from build123d import *

# Parameters (mm, degrees)
SKETCH1_R           = 17.5
BOSS_EXTRUDE1_DEPTH = 40


with BuildPart() as part:
    # Sketch1 → Boss-Extrude1 (new body)
    with BuildSketch(Plane.XY):
        Circle(SKETCH1_R)
        with BuildLine():
            ThreePointArc((-13.167433825, 7.184614567), (-13.858192988, 5.740251485), (-14.391071429, 4.230492068))
            ThreePointArc((-14.391071429, 4.230492068), (-12.25, 0), (-14.391071429, -4.230492068))
            ThreePointArc((-14.391071429, -4.230492068), (-13.858192988, -5.740251485), (-13.167433825, -7.184614567))
            ThreePointArc((-13.167433825, -7.184614567), (-8.66205807, -8.66205807), (-7.184614567, -13.167433825))
            ThreePointArc((-7.184614567, -13.167433825), (-5.740251485, -13.858192988), (-4.230492068, -14.391071429))
            ThreePointArc((-4.230492068, -14.391071429), (0, -12.25), (4.230492068, -14.391071429))
            ThreePointArc((4.230492068, -14.391071429), (5.740251485, -13.858192988), (7.184614567, -13.167433825))
            ThreePointArc((7.184614567, -13.167433825), (8.66205807, -8.66205807), (13.167433825, -7.184614567))
            ThreePointArc((13.167433825, -7.184614567), (13.858192988, -5.740251485), (14.391071429, -4.230492068))
            ThreePointArc((14.391071429, -4.230492068), (12.25, 0), (14.391071429, 4.230492068))
            ThreePointArc((14.391071429, 4.230492068), (13.858192988, 5.740251485), (13.167433825, 7.184614567))
            ThreePointArc((13.167433825, 7.184614567), (8.66205807, 8.66205807), (7.184614567, 13.167433825))
            ThreePointArc((7.184614567, 13.167433825), (5.740251485, 13.858192988), (4.230492068, 14.391071429))
            ThreePointArc((4.230492068, 14.391071429), (0, 12.25), (-4.230492068, 14.391071429))
            ThreePointArc((-4.230492068, 14.391071429), (-5.740251485, 13.858192988), (-7.184614567, 13.167433825))
            ThreePointArc((-7.184614567, 13.167433825), (-8.66205807, 8.66205807), (-13.167433825, 7.184614567))
        make_face(mode=Mode.SUBTRACT)
    extrude(amount=BOSS_EXTRUDE1_DEPTH)


solid = part.part
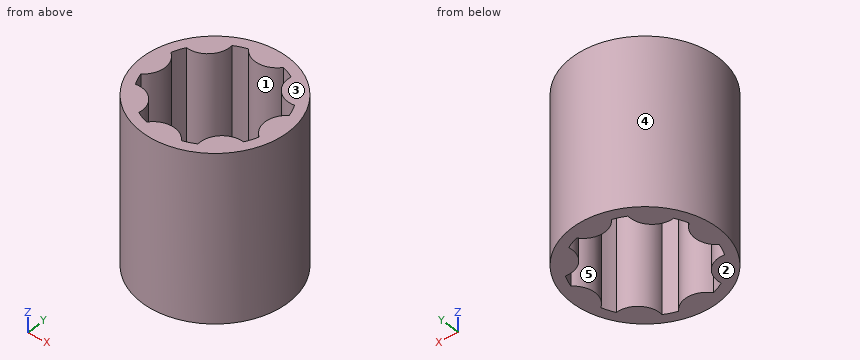
The model under review builds one solid part; all positions refer to its coordinate system, in mm. Face numbers are marked on the shaded views. A direction names the side the tool comes from. Give positions to 0.01 mm unless a question says otherwise; leave off trailing zeros. Write each loop counter-clockwise with the first axis right and the second up, starting at its lowest first coordinate (ties: lowest second). Pieces come first, ordered by that corner, then holes.
1. For P1, Ø2, axis at y = -7.5, z = 31, coming from the -X side; P2, Ø1.5, axis at y = 11, z = 16.5, coming from the -X side; P3, Ø6, axis at y = -8, z = 33.5, coming from the +X side, all flat-tipped, find the tip position at first contact; note any pin that passes through.
2. Add section D-D, the plane y = 15.5. Write out the cut boundary in (x, z).
3. Wall thickness on L1, parallel to Y at x = 13, z = 16; L2, parallel to Y at x = -10, z = 12; L3, parallel to X at y = -4.5, z = 36: over which ranges is each line inside the solid? List them lowest first.
4. Add section B-B, the plane y = 0. Write out the cut boundary in (x, z).
5. Tool access review of the marked faces 1 and 2: name each direction out of +Z, -Z, +X, -X, +Y, -Y from which nothing blocks a thin tool from reaching the whole face with its end or side.
6. Add section A-A, the plane z = 35. Write out the cut boundary in (x, y), plus the area to 3 significant figures.
7. Draft analysis for pull direction X (two halves, no side actions). For the marked faces 3, 4 and 5, state which applies: +X half, -X half, draft (parallel to the pull), parting line (faces both ways), or undercut.
Worked answers:
1. P1: stops at x = -16.25
1. P2: stops at x = -14.18
1. P3: stops at x = 16.77
2. outline: (-8.12, 0) - (8.12, 0) - (8.12, 40) - (-8.12, 40) - close
3. L1: y = -11.72 to -7.16, -2.7 to 2.7, 7.16 to 11.72
3. L2: y = -14.36 to -7.69, 7.69 to 14.36
3. L3: x = -16.91 to -14.31, 14.31 to 16.91
4. outline: (-17.5, 0) - (-12.25, 0) - (-12.25, 40) - (-17.5, 40) - close; (12.25, 0) - (17.5, 0) - (17.5, 40) - (12.25, 40) - close
5. face 1: +Z, -Z
5. face 2: -Z, +X, -X, +Y, -Y
6. outline: circle Ø35 at (0, 0); hole (-14.39, -4.23) arc R15 ccw to (-13.17, -7.18) arc R5.25 cw to (-7.18, -13.17) arc R15 ccw to (-4.23, -14.39) arc R5.25 cw to (4.23, -14.39) arc R15 ccw to (7.18, -13.17) arc R5.25 cw to (13.17, -7.18) arc R15 ccw to (14.39, -4.23) arc R5.25 cw to (14.39, 4.23) arc R15 ccw to (13.17, 7.18) arc R5.25 cw to (7.18, 13.17) arc R15 ccw to (4.23, 14.39) arc R5.25 cw to (-4.23, 14.39) arc R15 ccw to (-7.18, 13.17) arc R5.25 cw to (-13.17, 7.18) arc R15 ccw to (-14.39, 4.23) arc R5.25 cw to start
6. area: 384 mm2
7. face 3: draft
7. face 4: parting line
7. face 5: undercut
